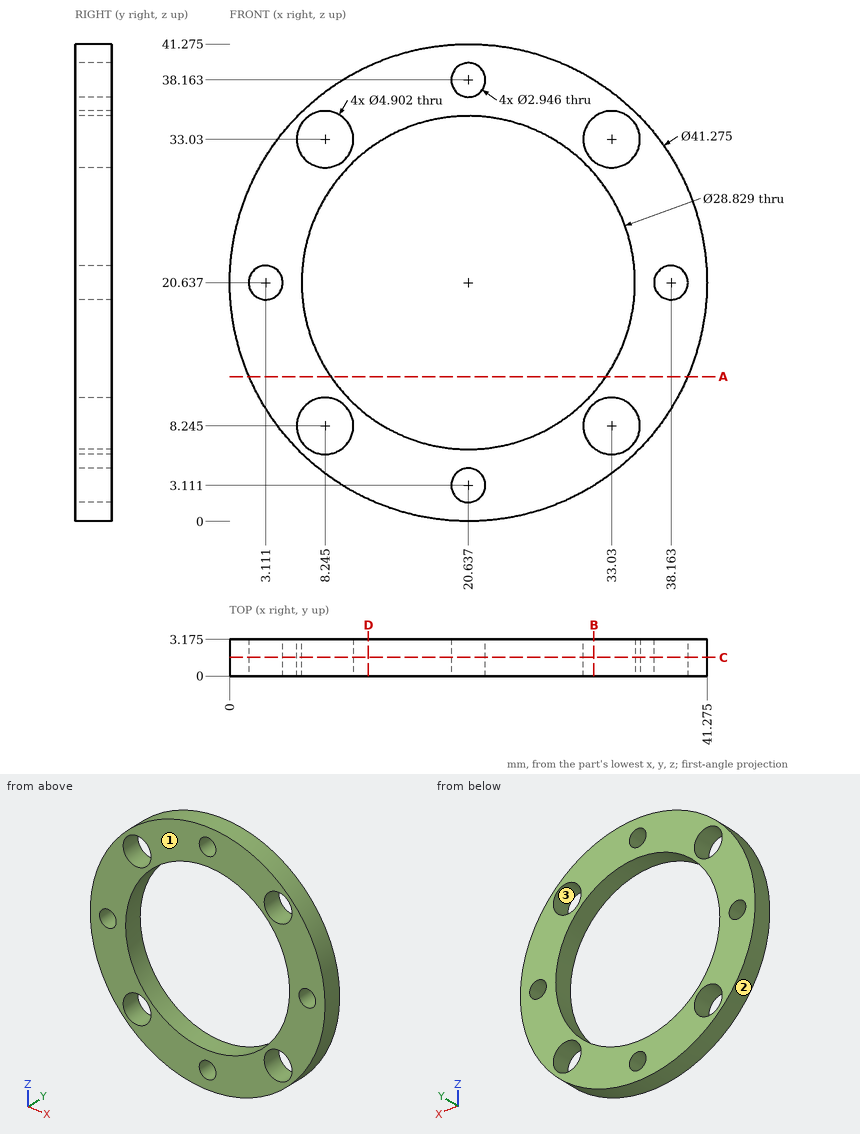
Could you check a few things on this drawing? It's one solid part, dimensions in mm from its lowest x, y, z. Round coordinates to 2 decimals unless told otherwise and drop trailing zeros. Write each loop counter-clockwise with the first axis right and the second up, starting at its lowest first coordinate (ties: lowest second). Pieces come first, ordered by that corner, then holes. Notation, with made-up numbers: (37, 25.25) -> (96, 25.25) arc R13 cw to (96, 44.25) -> close; hole circle Ø10 at (78.25, -9). An arc over 180 degrees is marked (long way). Use one line per item in the form item = value. Start each with the question number.
Q1. We'd pull the mould along Z, two halves only. Please class the marked faces 1, 2 and 3: +Z half, -Z half, draft (parallel to the pull), parting line (faces both ways), or undercut.
Q2. Imagine slicing it at D-D (x = 12). Please give me the cut outline in (y, z) (1 decimal).
Q3. If I drill on probe 1 along Z at (x, y) = (21, 2.8) (1 decimal); probe 2 along Z at (x, y) = (20, 1.4) (1 decimal); probe 3 along X at (y, z) = (1.5, 26) (1 decimal), over which ranges is the centre line in solid material (lowest first)? Write a range as [from, to].
Q4. Imagine slicing it at C-C (y = 1.6). Count the separate pieces of the cut face and the enclosed holes in it.
Q5. Imagine slicing it at B-B (x = 31.5). Please give me the cut outline in (y, z) (1 decimal).
Q6. Imagine slicing it at A-A (z = 12.5). Please give me the cut outline in (x, y) (1 decimal).
Q7. I'm going to push flat-ended pins straight in: P1, Ø4, axis at x = 33.03, z = 33.03, coming from the +Y side; P2, Ø1, axis at y = 2, z = 37, coming from the +X side. Where does each tip first touch, or does it pass through?
Worked out:
q1.face_1 = draft
q1.face_2 = parting line
q1.face_3 = undercut
q2.outline = (0, 1.9) -> (3.2, 1.9) -> (3.2, 9.1) -> (0, 9.1) -> close; (0, 32.2) -> (3.2, 32.2) -> (3.2, 39.4) -> (0, 39.4) -> close
q3.probe_1 = [0, 1.7], [4.5, 6.2], [35, 36.7], [39.6, 41.3]
q3.probe_2 = [0, 1.8], [4.4, 6.2], [35, 36.8], [39.5, 41.3]
q3.probe_3 = [0.7, 7.3], [34, 40.6]
q4.separate_pieces = 1
q4.enclosed_holes = 9
q5.outline = (0, 3.1) -> (3.2, 3.1) -> (3.2, 6.3) -> (0, 6.3) -> close; (0, 10.2) -> (3.2, 10.2) -> (3.2, 11.2) -> (0, 11.2) -> close; (0, 30.1) -> (3.2, 30.1) -> (3.2, 31.1) -> (0, 31.1) -> close; (0, 34.9) -> (3.2, 34.9) -> (3.2, 38.2) -> (0, 38.2) -> close
q6.outline = (1.7, 0) -> (8.7, 0) -> (8.7, 3.2) -> (1.7, 3.2) -> close; (32.5, 0) -> (39.6, 0) -> (39.6, 3.2) -> (32.5, 3.2) -> close
q7.P1 = through
q7.P2 = 33.84
